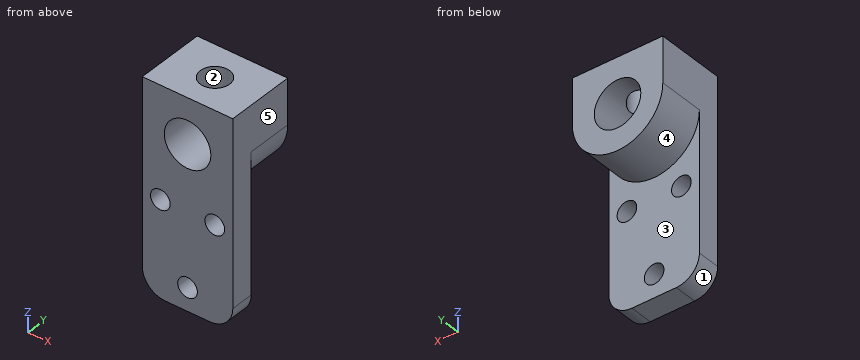
from build123d import *

# Parameters (mm, degrees)
SKETCH_1_W                = 12.446
SKETCH_1_H                = 28.448
EXTRUDE_1_DEPTH           = 9.525
CUT_EXTRUDE_1_DEPTH       = 6.35
HOLE_WIZARD_M2_5_1_D      = 2.7051
HOLE_WIZARD_M2_5_1_DEPTH  = 9.525
HOLE_WIZARD_M6_1_D        = 6.4008
HOLE_WIZARD_M3_5_1_REACH  = 48.703
HOLE_WIZARD_M3_5_1_BORE_R = 2.0193
FILLET_1_R                = 3.175


with BuildPart() as part:
    # 草图1 → 凸台-拉伸1 (new body)
    with BuildSketch(Plane(origin=(0, 36.5125, 0), x_dir=(1, 0, 0), z_dir=(0, 1, 0))):
        with Locations((0, 8.001)):
            Rectangle(SKETCH_1_W, SKETCH_1_H)
    extrude(amount=-EXTRUDE_1_DEPTH)

    # 草图2 → 切除-拉伸1 (cut)
    with BuildSketch(Plane(origin=(0, 36.5125, 0), x_dir=(-1, 0, 0), z_dir=(0, 1, 0))):
        with BuildLine():
            Line((6.223, -22.225), (6.223, 0))
            ThreePointArc((6.223, 0), (0, -6.223), (-6.223, 0))
            Line((-6.223, 0), (-6.223, -22.225))
            Line((-6.223, -22.225), (6.223, -22.225))
        make_face()
    extrude(amount=-CUT_EXTRUDE_1_DEPTH, mode=Mode.SUBTRACT)

    # M2.5 间隙孔1
    with Locations(Plane(origin=(0, 26.9875, 0), x_dir=(-1, 0, 0), z_dir=(0, -1, 0))):
        with Locations((-3.742261285, 9.034617948), (3.742261285, 9.034617948), (0, 19.05)):
            Hole(HOLE_WIZARD_M2_5_1_D / 2, depth=HOLE_WIZARD_M2_5_1_DEPTH)

    # M6 间隙孔1 (through all)
    with Locations(Plane(origin=(0, 36.5125, 0), x_dir=(1, 0, 0), z_dir=(0, 1, 0))):
        with Locations((0, 0)):
            Hole(HOLE_WIZARD_M6_1_D / 2)

    # M3.5 间隙孔1 bore → M3.5 间隙孔1 (cut, up to next)
    with BuildSketch(Plane.XY.offset(6.223), mode=Mode.PRIVATE) as hole_wizard_m3_5_1_sk1:
        with Locations((0, 31.75)):
            Circle(HOLE_WIZARD_M3_5_1_BORE_R)
    hole_wizard_m3_5_1_tool1 = extrude(hole_wizard_m3_5_1_sk1.sketch, amount=-HOLE_WIZARD_M3_5_1_REACH, mode=Mode.PRIVATE) & part.part
    add(hole_wizard_m3_5_1_tool1.solids().sort_by_distance((0, 31.75, 6.223))[0], mode=Mode.SUBTRACT)

    # 圆角1
    fillet_1_edges = [part.edges().sort_by_distance(p)[0] for p in [
        (-6.223, 28.575, -22.225),
        (6.223, 28.575, -22.225),
    ]]
    fillet(fillet_1_edges, radius=FILLET_1_R)


solid = part.part
The listing builds one solid part. Answer for the finished solid, in the listing's coordinates (mm). Face numbers are marked on the shaded views. A direction names the side the tool comes from. Round coordinates to 2 decimals unless told otherwise and drop trailing zeros. Order: outer loops, then holes, each group sorted by start corner. A loop starts at its lowest first (then second) coordinate and runs counter-clockwise, first axis right, second up. Notation, with made-up numbers: (67, 48) - (92, 48) arc R26 ccw to (92, 62) - close; hole circle Ø6 at (-4, 47). An arc over 180 degrees is marked (long way). Write item = value, one per line. Start each with the question number.
1) Section C-C, the plane z = -18 is taken. Write down the section's boundary in (x, y), plus the area to 3 significant figures.
2) For a pull along Y with two mould halves and no side action, classify the marked faces 1, 2 and 3 as released by +Y, released by -Y, zero draft, split by the parting line, or undercut.
3) Section B-B, the plane y = 34.75 is taken. Write down the section's boundary in (x, z), plus the area to 3 significant figures.
4) Straight lines are drawn through the part: L1, parallel to Z at x = 0, y = 28.5 (3 decimals); L2, parallel to X at y = 31.75, z = 4.6; L3, parallel to Y at x = 0, z = 4.7. For each, find the intervals that lie inside material, in ascending order.
5) For the marked faces 4 and 5, determine the directions among +Z, -Z, +X, -X, +Y, -Y from which every point of the face is accessible in a straight line to the end or side of a thin tool.
6) Given pin 1 (2.5 mm diameter, centred on x = 0, y = 31.75, fed in from -Z); pin 2 (3 mm diameter, centred on x = -3.74, z = -9.03, fed in from +Y); pin 3 (5 mm diameter, centred on x = 0, y = 31, fed in from +Z); pin 4 (1 mm diameter, centred on y = 35.5, z = -2, fed in from -X), each flat-ended and moving along its own axis, determine where each tip first touches the part or whether it passes through.
7) Section A-A, the plane x = -0.5 is taken. Write down the section's boundary in (y, z) (1 decimal).
8) Section D-D, the plane x = 4.5 is taken. Write down the section's boundary in (y, z).
Results list:
q1.outline = (-6.22, 26.99) - (-0.85, 26.99) - (-0.85, 30.16) - (-6.22, 30.16) - close; (0.85, 26.99) - (6.22, 26.99) - (6.22, 30.16) - (0.85, 30.16) - close
q1.area = 34.1 mm^2
q2.face_1 = zero draft
q2.face_2 = undercut
q2.face_3 = released by +Y
q3.outline = (-6.22, 0) arc R6.22 ccw to (6.22, 0) - (6.22, 6.22) - (-6.22, 6.22) - close; hole circle Ø6.4 at (0, 0)
q3.area = 106 mm^2
q4.L1 = -22.225 to -20.403, -17.697 to -3.2, 3.2 to 6.223
q4.L2 = -6.22 to -2.02, 2.02 to 6.22
q4.L3 = 26.99 to 29.73, 33.77 to 36.51
q5.face_4 = -Z, +Y
q5.face_5 = +Z, -Z, +X, +Y, -Y
q6.pin_1 = -6.22
q6.pin_2 = 30.16
q6.pin_3 = 6.22
q6.pin_4 = -6.04
q7.outline = (27, -22.2) - (30.2, -22.2) - (30.2, -20.3) - (27, -20.3) - close; (27, -17.8) - (30.2, -17.8) - (30.2, -6.2) - (36.5, -6.2) - (36.5, -3.2) - (27, -3.2) - close; (27, 3.2) - (29.8, 3.2) - (29.8, 6.2) - (27, 6.2) - close; (33.7, 3.2) - (36.5, 3.2) - (36.5, 6.2) - (33.7, 6.2) - close
q8.outline = (26.99, -21.87) - (30.16, -21.87) - (30.16, -10.15) - (26.99, -10.15) - close; (26.99, -7.91) - (30.16, -7.91) - (30.16, -4.3) - (36.51, -4.3) - (36.51, 6.22) - (26.99, 6.22) - close
